The model under review builds one solid part; all positions refer to its coordinate system, in mm. A direction names the side the tool comes from. Round coordinates to 2 decimals unless told otherwise and drop trailing zeros. Order: outer loops, then holes, each group sorted by start corner. A loop starts at its lowest first (then second) coordinate and runs counter-clockwise, first axis right, second up.
```python
from build123d import *

# Parameters (mm, degrees)
BOSS_EXTRUDE1_DEPTH   = 55.6
SKETCH1_R             = 9.65
BOSS_EXTRUDE1_2_DEPTH = 55.6
BOSS_EXTRUDE1_3_DEPTH = 55.6
SKETCH2_W             = 54.5
SKETCH2_H             = 19.3
BOSS_EXTRUDE2_DEPTH   = 8
SKETCH3_W             = 54.5
SKETCH3_H             = 19.3
BOSS_EXTRUDE3_DEPTH   = 8


with BuildPart() as part:
    # Sketch1 → Boss-Extrude1 (new body)
    with BuildSketch(Plane(origin=(0, 0, 0), x_dir=(1, 0, 0), z_dir=(0, 1, 0))):
        with BuildLine():
            Line((-17.574982219, 9.65), (-27.25, 9.65))
            Line((-27.25, 9.65), (-27.25, -9.65))
            Line((-27.25, -9.65), (-17.574982219, -9.65))
            ThreePointArc((-17.574982219, -9.65), (-20.05, 0), (-17.574982219, 9.65))
        make_face()
    extrude(amount=BOSS_EXTRUDE1_DEPTH)



with BuildPart() as body_2:
    # Sketch1 → Boss-Extrude1 2 (new body)
    with BuildSketch(Plane(origin=(0, 0, 0), x_dir=(1, 0, 0), z_dir=(0, 1, 0))):
        Circle(SKETCH1_R)
    extrude(amount=BOSS_EXTRUDE1_2_DEPTH)


with BuildPart() as body_3:
    # Sketch1 → Boss-Extrude1 3 (new body)
    with BuildSketch(Plane(origin=(0, 0, 0), x_dir=(1, 0, 0), z_dir=(0, 1, 0))):
        with BuildLine():
            Line((27.25, 9.65), (17.574982219, 9.65))
            ThreePointArc((17.574982219, 9.65), (19.421391473, 4.981169868), (20.05, 0))
            ThreePointArc((20.05, 0), (19.421391473, -4.981169868), (17.574982219, -9.65))
            Line((17.574982219, -9.65), (27.25, -9.65))
            Line((27.25, -9.65), (27.25, 9.65))
        make_face()
    extrude(amount=BOSS_EXTRUDE1_3_DEPTH)


with BuildPart() as part_1:
    add(part.part)

    add(body_2.part)  # Boss-Extrude2 merges body 2

    add(body_3.part)  # Boss-Extrude2 merges body 3
    # Sketch2 → Boss-Extrude2 (add)
    with BuildSketch(Plane(origin=(0, 55.6, 0), x_dir=(1, 0, 0), z_dir=(0, 1, 0))):
        Rectangle(SKETCH2_W, SKETCH2_H)
    extrude(amount=-BOSS_EXTRUDE2_DEPTH)

    # Sketch3 → Boss-Extrude3 (add)
    with BuildSketch(Plane.XZ):
        Rectangle(SKETCH3_W, SKETCH3_H)
    extrude(amount=-BOSS_EXTRUDE3_DEPTH)


solid = part_1.part
```
(1) For faces 4 (the flat face through (-18, 27, -9.65)), 5 (the cylindrical face through (9.204, 27.523, -2.899)), list the 3-axis set-ups (+Z, -Z, +X, -X, +Y, -Y) from which the entire face can be reached by the end or side of a thin tool; tool diameter is ignored.
Data:
face 4: -Z, +X, -X, +Y, -Y
face 5: none
(2) Consider section B-B (y = 41). Write out the cut boundary in (x, z), and give its area (3 significant figures).
Data:
outline: (-27.25, -9.65) - (-17.57, -9.65) arc R20.05 cw to (-17.57, 9.65) - (-27.25, 9.65) - close; circle Ø19.3 at (0, 0); (17.57, -9.65) - (27.25, -9.65) - (27.25, 9.65) - (17.57, 9.65) arc R20.05 cw to start
area: 601 mm2
(3) Consider section C-C (z = -6.5). Write out the cut boundary in (x, y).
Data:
outline: (-27.25, 0) - (27.25, 0) - (27.25, 55.6) - (-27.25, 55.6) - close; hole (-18.97, 8) - (-7.13, 8) - (-7.13, 47.6) - (-18.97, 47.6) - close; hole (7.13, 8) - (18.97, 8) - (18.97, 47.6) - (7.13, 47.6) - close
(4) Insertion check: pin 1 (3 mm diameter, centred on x = -8, y = 11, fed in from +Z); pin 2 (5 mm diameter, centred on x = 11, y = 40, fed in from +Z). Each pin has a flat end and moves straight along its axis. Give the tip position at first contact, or say it passes through.
Data:
pin 1: stops at z = 7.13
pin 2: stops at z = 4.57
(5) To check wall thickness, follow probe 1 along Y at (x, z) = (-8, -8.25); probe 2 along X at (y, z) = (46, 6); probe 3 along X at (y, z) = (14.5, 2.25). State the ranges of each line that lie inside material, in increasing order.
Data:
probe 1: y = 0 to 8, 47.6 to 55.6
probe 2: x = -27.25 to -19.13, -7.56 to 7.56, 19.13 to 27.25
probe 3: x = -27.25 to -19.92, -9.38 to 9.38, 19.92 to 27.25
(6) Draft analysis for pull direction Y (two halves, no side actions). For faces 1 (the flat face through (0, 55.6, 0)), 2 (the flat face through (14, 8, 0)), 3 (the flat face through (-27.25, 27, 0)), state which applies: pulls with the +Y half, pulls with the -Y half, needs draft (parallel to the pull), parting line crosses it, or undercut.
Data:
face 1: pulls with the +Y half
face 2: undercut
face 3: needs draft
(7) Consider section A-A (x = 16). Write out the cut boundary in (y, z).
Data:
outline: (0, -9.65) - (8, -9.65) - (8, 9.65) - (0, 9.65) - close; (47.6, -9.65) - (55.6, -9.65) - (55.6, 9.65) - (47.6, 9.65) - close
